Verification items for the finished model (mm, model axes). A direction names the side the tool comes from. Give positions to 0.01 mm unless a question says otherwise; leave off trailing zeros. Write each loop counter-clockwise with the first axis right and the second up, starting at its lowest first coordinate (ties: lowest second). Pieces come first, ordered by that corner, then holes.
from build123d import *

# Parameters (mm, degrees)
F1_DEPTH = 50.8


with BuildPart() as f1:
    # F0 (on Front) → F1 (new body)
    with BuildSketch(Plane.XZ):
        Polygon((-38.1, 0), (0, 0), (0, 12.7), (-1.27, 12.7), (-2.194484, 10.16), (-3.464484, 10.16), (-4.734484, 11.43), (-6.004484, 10.16), (-7.274484, 10.16), (-8.544484, 11.43), (-9.814484, 10.16), (-11.084484, 10.16), (-12.354484, 11.43), (-13.624484, 10.16), (-14.894484, 10.16), (-16.164484, 11.43), (-17.434484, 10.16), (-18.704484, 10.16), (-19.974484, 11.43), (-21.244484, 10.16), (-22.514484, 10.16), (-23.784484, 11.43), (-25.054484, 10.16), (-25.4, 10.16), (-25.4, 50.8), (-38.1, 50.8), align=None)
    extrude(amount=-F1_DEPTH)


solid = f1.part
Item 1: Sectioned sample at B-B on z = 16. Record the cut outline in (x, y).
Answer key:
outline: (-38.1, 0) - (-25.4, 0) - (-25.4, 50.8) - (-38.1, 50.8) - close
Item 2: Set-up check for faces 4 (the face through (-9.171, 25.044, 10.804)), 5 (the face through (-19, 25, 0)): record each of +Z, -Z, +X, -X, +Y, -Y from which the full face is reachable in a straight line by a thin tool's end or side.
Answer key:
face 4: +Z, +Y, -Y
face 5: -Z, +X, -X, +Y, -Y
Item 3: Sectioned sample at A-A on y = 36.5. Record the cut outline in (x, z), then the cut area to 3 significant figures.
Answer key:
outline: (-38.1, 0) - (0, 0) - (0, 12.7) - (-1.27, 12.7) - (-2.19, 10.16) - (-3.46, 10.16) - (-4.73, 11.43) - (-6, 10.16) - (-7.27, 10.16) - (-8.54, 11.43) - (-9.81, 10.16) - (-11.08, 10.16) - (-12.35, 11.43) - (-13.62, 10.16) - (-14.89, 10.16) - (-16.16, 11.43) - (-17.43, 10.16) - (-18.7, 10.16) - (-19.97, 11.43) - (-21.24, 10.16) - (-22.51, 10.16) - (-23.78, 11.43) - (-25.05, 10.16) - (-25.4, 10.16) - (-25.4, 50.8) - (-38.1, 50.8) - close
area: 917 mm2
Item 4: Release check for a two-part mould opening along X. For faces 1 (the face through (0, 25, 6)), 2 (the face through (-12.981, 25.044, 10.804)), 3 (the face through (-1, 25, 12.7)) record: released by +X, released by -X, zero draft, split by the parting line, or undercut.
Answer key:
face 1: released by +X
face 2: undercut
face 3: zero draft
Item 5: Scan lines: line 1 along X through (y, z) = (36, 39); line 2 along Z through (x, y) = (-21.5, 39); line 3 along X through (y, z) = (46.5, 11.5). Record each from-to range of solid material in increasing order.
Answer key:
line 1: x = -38.1 to -25.4
line 2: z = 0 to 10.16
line 3: x = -38.1 to -25.4, -1.71 to 0
Item 6: Depth check by flat-ended pin: pin 1 (1 mm diameter, centred on x = -3, y = 28, fed in from +Z); pin 2 (1.4 mm diameter, centred on x = -18.5, y = 37.5, fed in from +Z); pin 3 (5 mm diameter, centred on y = 27.5, z = 32, fed in from +X); pin 4 (10 mm diameter, centred on x = -5, y = 44.5, fed in from -Z). Enter the tip coordinate at first touch or a pass-through.
Answer key:
pin 1: stops at z = 10.2
pin 2: stops at z = 10.66
pin 3: stops at x = -25.4
pin 4: stops at z = 0
